Can you work these out from the model? Positions are in its coordinate system, mm. Face numbers are marked on the shaded views. A direction names the side the tool comes from. Give positions to 0.01 mm unless a question says otherwise; leave off trailing zeros. Write each loop counter-clockwise with the first axis right and the second up, starting at its lowest first coordinate (ties: lowest second). Pieces come first, ordered by that corner, then holes. Notation, with made-up numbers: M -13,59.5 L 33,59.5 A25 ccw 33,74.5 Z; hole C 10,8 d5. An arc over 180 degrees is marked long. Write each question's results on one line, items separated by ' | '.
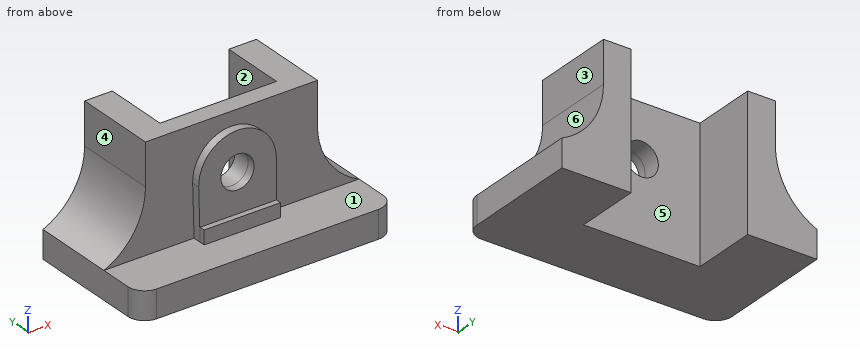
from build123d import *

# Parameters (mm, degrees)
F2_DEPTH    = 10
F3_DEPTH    = 48
F4_R        = 6
F5_DEPTH    = 3
F6_W        = 27.4810515978
F6_H        = 5
F7_DEPTH    = 2
F8_DEPTH    = 20
F9_T1_DEPTH = 30.1119658546
F10_R       = 6


# Not quite as in the source:
# - a fillet or chamfer that OpenCascade refuses, or shapes differently, is made with other operations: its cross-section is extruded or revolved along the edge and cut away or added


with BuildPart() as f2:
    # F0 (on Top) → F2 (new body)
    with BuildSketch(Plane.XY):
        Polygon((46, -18), (46, 30), (31, 30), (31, -0.1119658546), (-31, -0.1119658546), (-31, 30), (-46, 30), (-46, -18), align=None)
        Polygon((31, -0.1119658546), (31, 30), (21, 30), (21, 6.4026141707), (-21, 6.4026141707), (-21, 30), (-31, 30), (-31, -0.1119658546), align=None)
    extrude(amount=F2_DEPTH)

    # F1 (on Top) → F3 (join)
    with BuildSketch(Plane.XY):
        Polygon((31, -0.1119658546), (31, 30), (21, 30), (21, 6.4026141707), (-21, 6.4026141707), (-21, 30), (-31, 30), (-31, -0.1119658546), align=None)
    extrude(amount=F3_DEPTH)

    # F4 (on face) → F5 (join)
    with BuildSketch(Plane.XZ.offset(0.1119658546)):
        with BuildLine():
            Line((14, 10), (14, 29))
            ThreePointArc((14, 29), (-0.1930996384, 42.9986682413), (-13.9946732185, 28.6138374607))
            Line((-13.9946732185, 28.6138374607), (-13.4810515978, 10))
            Line((-13.4810515978, 10), (14, 10))
        make_face()
        with Locations((0, 29)):
            Circle(F4_R, mode=Mode.SUBTRACT)
    extrude(amount=F5_DEPTH)

    # F6 (on face) → F7 (join)
    with BuildSketch(Plane.XZ.offset(3.1119658546)):
        with Locations((0.2594742011, 12.5)):
            Rectangle(F6_W, F6_H)
    extrude(amount=F7_DEPTH)

    # F8 (cut): a face of the model
    f8_faces = [f2.faces().sort_by_distance(p)[0] for p in [
        (0, -0.1119658546, 29),
    ]]
    extrude(f8_faces, amount=-F8_DEPTH, mode=Mode.SUBTRACT)

    # F9: fillet of radius 25 on 2 edges, made by hand

    # F9_s2 → F9_t1 (join)
    with BuildSketch(Plane.XZ.offset(-30)):
        with BuildLine():
            ThreePointArc((46, 10), (35.0834993366, 19.2198145372), (31, 32.9128784748))
            Line((31, 32.9128784748), (31, 10))
            Line((31, 10), (46, 10))
        make_face()
        with BuildLine():
            ThreePointArc((-46, 10), (-35.0834993366, 19.2198145372), (-31, 32.9128784748))
            Line((-31, 32.9128784748), (-31, 10))
            Line((-31, 10), (-46, 10))
        make_face()
    extrude(amount=F9_T1_DEPTH)

    # F10
    f10_edges = [f2.edges().sort_by_distance(p)[0] for p in [
        (-46, -18, 5),
        (46, -18, 5),
    ]]
    fillet(f10_edges, radius=F10_R)


solid = f2.part
Item 1: For the marked faces 5 and 6, which set-ups out of +Z, -Z, +X, -X, +Y, -Y let a thin tool reach every point of the face, with its end or its side?
Geometry says:
face 5: +Z, -Z, +Y | face 6: +Z, +X, +Y, -Y
Item 2: I'm going to push flat-ended pins straight in: pin 1 (12 mm diameter, centred on y = 15.5, z = 42.5, fed in from -X); pin 2 (4 mm diameter, centred on y = -1.5, z = 16, fed in from +X); pin 3 (19 mm diameter, centred on y = 14, z = 35.5, fed in from +X). Where does each tip first touch, or does it pass through?
Geometry says:
pin 1: stops at x = -31 | pin 2: stops at x = 39.02 | pin 3: stops at x = 31.97
Item 3: If I drill on line 1 (X direction, y = 7, z = 8); line 2 (Z direction, x = 0, y = 3); line 3 (X direction, y = 16.5, z = 33), over which ranges is the centre line in solid material (lowest first)? Write a range as from..to.
Geometry says:
line 1: x = -46..-21, 21..46 | line 2: z = 0..23, 35..48 | line 3: x = -31..-21, 21..31
Item 4: I want a section at D-D, the plane z = 4. Please give me the cut outline in (x, y), and give its area (3 significant figures).
Geometry says:
outline: M -46,-12 A6 ccw -40,-18 L 40,-18 A6 ccw 46,-12 L 46,30 L 21,30 L 21,6.4 L -21,6.4 L -21,30 L -46,30 Z | area: 3,410 mm2
Item 5: Thinking about a two-plate mould opening in X: for the marked faces 1, 2, 3 and 4, which applies, +X half, -X half, draft (parallel to the pull), parting line (faces both ways), or undercut?
Geometry says:
face 1: draft | face 2: undercut | face 3: +X half | face 4: -X half
Item 6: I want a section at C-C, the plane y = 15.5. Please give me the cut outline in (x, z).
Geometry says:
outline: M -46,0 L -21,0 L -21,48 L -31,48 L -31,32.91 A25 cw -46,10 Z; M 21,0 L 46,0 L 46,10 A25 cw 31,32.91 L 31,48 L 21,48 Z
Item 7: I want a section at B-B, the plane x = 0. Please give me the cut outline in (y, z).
Geometry says:
outline: M -18,0 L 6.4,0 L 6.4,23 L -3.11,23 L -3.11,15 L -5.11,15 L -5.11,10 L -18,10 Z; M -3.11,35 L 6.4,35 L 6.4,48 L -0.11,48 L -0.11,43 L -3.11,43 Z
Item 8: I want a section at A-A, the plane y = 5. Please give me the cut outline in (x, z), and give its area (3 significant figures).
Geometry says:
outline: M -46,0 L 46,0 L 46,10 A25 cw 31,32.91 L 31,48 L -31,48 L -31,32.91 A25 cw -46,10 Z; hole C 0,29 d12 | area: 3,350 mm2
